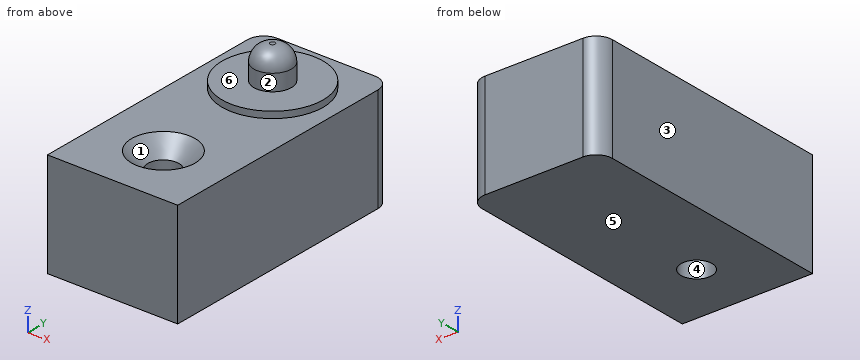
```python
from build123d import *

# Parameters (mm, degrees)
F0_R     = 1.2065
F1_DEPTH = 8.128
F2_SIZE  = 1.27
F3_R     = 3.937
F4_DEPTH = 0.508
F5_R     = 1.4605
F6_DEPTH = 2.54
F7_R     = 1.27


with BuildPart() as f1:
    # F0 (on Top) → F1 (new body)
    with BuildSketch(Plane.XY):
        with BuildLine():
            Line((-5.08, -10.16), (5.08, -10.16))
            Line((5.08, -10.16), (5.08, 8.89))
            ThreePointArc((5.08, 8.89), (4.708026, 9.788026), (3.81, 10.16))
            Line((3.81, 10.16), (-3.81, 10.16))
            ThreePointArc((-3.81, 10.16), (-4.708026, 9.788026), (-5.08, 8.89))
            Line((-5.08, 8.89), (-5.08, -10.16))
        make_face()
        with Locations((0, -5.3213)):
            Circle(F0_R, mode=Mode.SUBTRACT)
    extrude(amount=F1_DEPTH)

    # F2
    f2_edges = [f1.edges().sort_by_distance(p)[0] for p in [
        (-1.2065, -5.3213, 8.128),
    ]]
    chamfer(f2_edges, length=F2_SIZE)

    # F3 (on face) → F4 (join)
    with BuildSketch(Plane.XY.offset(8.128)):
        with Locations((0, 5.08)):
            Circle(F3_R)
    extrude(amount=F4_DEPTH)

    # F5 (on face) → F6 (join)
    with BuildSketch(Plane.XY.offset(8.636)):
        with Locations((0, 5.08)):
            Circle(F5_R)
    extrude(amount=F6_DEPTH)

    # F7
    f7_edges = [f1.edges().sort_by_distance(p)[0] for p in [
        (-1.4605, 5.08, 11.176),
    ]]
    fillet(f7_edges, radius=F7_R)


solid = f1.part
```
For this review, take the finished solid that the model builds, in its own axes (mm). Face numbers are marked on the shaded views. A direction names the side the tool comes from. Coordinates: 2 decimals unless noted, no trailing zeros. Write each loop counter-clockwise with the first axis right and the second up, starting at its lowest first coordinate (ties: lowest second). Pieces come first, ordered by that corner, then holes.
(1) Tool access review of the marked faces 5 and 6: name each direction out of +Z, -Z, +X, -X, +Y, -Y from which nothing blocks a thin tool from reaching the whole face with its end or side.
(2) For pin 1 Ø4 at (x, y) = (-1, -6) entering from +Z; pin 2 Ø1.5 at (x, y) = (3, 2.5) entering from +Z; pin 3 Ø1.4 at (x, y) = (0, -5.32) entering from +Z, all flat-tipped, find the tip position at first contact; note any pin that passes through.
(3) Add section B-B on z = 9.5. Give the boundary of the cut face in (x, y), then the cut area to 3 significant figures.
(4) Add section A-A on x = -3.25. Give the boundary of the cut face in (y, z).
(5) The part is to be moulded in two halves that separate along X. For the marked faces 1, 2, 3 and 4, say which applies: +X half, -X half, draft (parallel to the pull), parting line (faces both ways), or undercut.
(6) Add section C-C on z = 3.5. Give the boundary of the cut face in (x, y).
(7) Wall thickness on probe 1 along Y at (x, z) = (0, 1.75); probe 2 along Z at (x, y) = (0, -1.5); probe 3 along Z at (x, y) = (0.5, 1.75): over which ranges is each line inside the solid? List them lowest first.
Answer sheet:
1. face 5: -Z, +X, -X, +Y, -Y
1. face 6: +Z
2. pin 1: stops at z = 8.13
2. pin 2: stops at z = 8.64
2. pin 3: passes through
3. outline: circle Ø2.92 at (0, 5.08)
3. area: 6.70 mm2
4. outline: (-10.16, 0) - (10.16, 0) - (10.16, 8.13) - (7.3, 8.13) - (7.3, 8.64) - (2.86, 8.64) - (2.86, 8.13) - (-10.16, 8.13) - close
5. face 1: undercut
5. face 2: parting line
5. face 3: -X half
5. face 4: undercut
6. outline: (-5.08, -10.16) - (5.08, -10.16) - (5.08, 8.89) arc R1.27 ccw to (3.81, 10.16) - (-3.81, 10.16) arc R1.27 ccw to (-5.08, 8.89) - close; hole circle Ø2.41 at (0, -5.32)
7. probe 1: y = -10.16 to -6.53, -4.11 to 10.16
7. probe 2: z = 0 to 8.13
7. probe 3: z = 0 to 8.64
